Build history of the part. All positions in model axes, mm. Face numbers are marked on the shaded views. A direction names the side the tool comes from. Round coordinates to 2 decimals unless told otherwise and drop trailing zeros. Write each loop counter-clockwise with the first axis right and the second up, starting at its lowest first coordinate (ties: lowest second). Pieces come first, ordered by that corner, then holes.
Item 1: 3-axis set-ups, long thin cutter, end or side, ignore diameter. For the marked faces 4 and 5: which of +Z, -Z, +X, -X, +Y, -Y reach the whole face in a straight line?
Item 2: Mould opens along X. For the marked faces 1, 2 and 3 say: +X half, -X half, draft (parallel to the pull), parting line (faces both ways), or undercut.
Item 3: Band-saw the part on A-A, the plane z = -11. Write the cut outline in (x, y).
Item 4: Band-saw the part on B-B, the plane y = 40.5. Write the cut outline in (x, z).
Item 5: Drop flat-ended pins along their axis: pin 1 Ø1.5 at (x, y) = (-27, 33.5) entering from -Z; pin 2 Ø4 at (x, y) = (-7.5, 49) entering from +Z; pin 3 Ø6 at (x, y) = (-21, 21.5) entering from +Z. Give the stop position or say it passes through.
Item 6: Wall check: probe 1 along X at (y, z) = (30, -9.5); probe 2 along Y at (x, z) = (-29.5, -1.95); probe 3 along Y at (x, z) = (-18.5, -2.5). Give the ranges that are in metal, low to high.
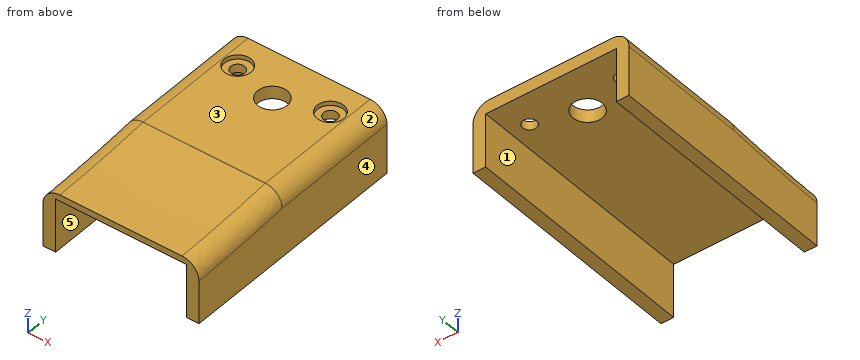
Autodesk Inventor part; units mm, degrees
ref_plane "YZ Plane" through (0, 0, 0) normal (1, 0, 0) x (0, 1, 0)
ref_plane "XZ Plane" through (0, 0, 0) normal (0, 1, 0) x (-1, 0, 0)
ref_plane "XY Plane" through (0, 0, 0) normal (0, 0, 1) x (1, 0, 0)
sketch "Esquisse1" plane through (0, 0, 0) normal (0, 1, 0) x (-1, 0, 0)
  line L0 (0, 0) -> (37, 0)
  line L1 (37, 0) -> (37, -31.5)
  line L2 (37, -31.5) -> (0, -31.5)
  line L3 (0, -31.5) -> (0, 0)
  line L4 (34, -28.5) -> (34, -3)
  line L5 (34, -3) -> (3, -3)
  line L6 (3, -3) -> (3, -28.5)
  line L7 (3, -28.5) -> (34, -28.5)
  line L8 (3, -15.75) -> (0, -15.75)
  line L9 (34, -15.75) -> (37, -15.75)
  dimension "d0" = 3
  dimension "d1" = 31
  dimension "d2" = 25.5
extrude "Extrusion1" add sketch "Esquisse1" along normal blind 56.5 contours L0 L1 L9 L4 L5 L6 L8 L3
sketch "Esquisse2" plane through (-37, 0, 0) normal (0, 0, 1) x (1, 0, 0)
  line L0 (7.5, 49) -> (29.5, 49) construction
  circle A0 centre (7.5, 49) radius 1.65
  circle A1 centre (29.5, 49) radius 1.65
  line L1 (34, 0) -> (3, 0) construction
  line L2 (18.5, 0) -> (18.5, 49) construction
  point P0 (37, 0)
  dimension "d5" = 3.3
  dimension "d6" = 49
  dimension "d7" = 22
extrude "Extrusion2" cut sketch "Esquisse2" against normal through all
sketch "Esquisse3" plane through (-33, 0, 0) normal (0, 0, 1) x (1, 0, 0)
  line L0 (-4, 56.5) -> (33, 56.5) construction
  line L1 (-4, 0) -> (33, 0) construction
  circle A0 centre (3.5, 49) radius 1.65 construction
  circle A1 centre (25.5, 49) radius 1.65 construction
  circle A2 centre (3.5, 49) radius 1.65 construction
  circle A3 centre (3.5, 49) radius 3.15
  circle A4 centre (25.5, 49) radius 3.15
  line L2 (33, 0) -> (33, 56.5)
  line L3 (-4, 0) -> (-4, 56.5)
  dimension "d11" = 6.3
extrude "Extrusion3" cut sketch "Esquisse3" against normal blind 1
sketch "Esquisse4" plane through (-33, 0, 0) normal (0, 0, 1) x (1, 0, 0)
  line L0 (-4, 56.5) -> (33, 56.5) construction
  line L1 (14.5, 56.5) -> (14.5, 0) construction
  line L2 (30, 0) -> (-1, 0) construction
  circle A0 centre (14.5, 45.5) radius 3.5
  point P0 (33, 0)
  point P1 (0, 56.5)
  point P2 (29, 56.5)
  dimension "d14" = 45.5
  dimension "d15" = 7
extrude "Extrusion4" cut sketch "Esquisse4" against normal through all
sketch "Esquisse5" plane through (0, 0, 0) normal (1, 0, 0) x (0, 0, -1)
  line L0 (0, 0) -> (1.5, 0)
  line L1 (0, 0) -> (15.75, 0)
  line L2 (0, 0) -> (0, 56.5)
  spline S0 degree 2 poles (1.5, 0) (1.2491, 12.5149) (0, 25) knots 0 0 0 1 1 1
  line L3 (0, 25) -> (0, 0)
  point P0 (1, 12.5)
  dimension "d18" = 1.5
  dimension "d19" = 25
  dimension "d20" = 12.5
  dimension "d21" = 1
extrude "Extrusion5" cut sketch "Esquisse5" against normal through all
fillet "Congé2" radius 4 4 edges at (0, 12.5075, -0.9996) (0, 40.75, 0) (-37, 40.75, 0) (-37, 12.5149, -0.9991)
fillet "Congé3" radius 1 3 edges at (-18.5, 25, 0) (-1.1716, 25, -1.1716) (-35.8284, 25, -1.1716)
properties part number "part1_top"
Results:
1. face 4: +Z, -Z, +X, +Y, -Y
1. face 5: -Z, +Y, -Y
2. face 1: undercut
2. face 2: +X half
2. face 3: draft
3. outline: (-37, 0) - (-34, 0) - (-34, 56.5) - (-37, 56.5) - close; (-3, 0) - (0, 0) - (0, 56.5) - (-3, 56.5) - close
4. outline: (-37, -15.75) - (-34, -15.75) - (-34, -3) - (-3, -3) - (-3, -15.75) - (0, -15.75) - (0, -4) arc R4 ccw to (-4, 0) - (-33, 0) arc R4 ccw to (-37, -4) - close
5. pin 1: stops at z = -3
5. pin 2: stops at z = -1
5. pin 3: stops at z = -0.05
6. probe 1: x = -37 to -34, -3 to 0
6. probe 2: y = 0 to 47.35, 50.65 to 56.5
6. probe 3: y = 0 to 42, 49 to 56.5
